```python
from build123d import *

# Parameters (mm, degrees)
SKETCH1_R            = 25
BOSS_EXTRUDE2_DEPTH  = 3
SKETCH3_R            = 57
BOSS_EXTRUDE10_DEPTH = 2
SKETCH8_R            = 51
SKETCH8_R_2          = 45
BOSS_EXTRUDE11_DEPTH = 6
SKETCH9_R            = 10
BOSS_EXTRUDE12_DEPTH = 6
SKETCH10_R           = 57
BOSS_EXTRUDE13_DEPTH = 2
FILLET1_R            = 2
FILLET2_R            = 2
FILLET3_R            = 2
FILLET4_R            = 2
SKETCH11_R           = 50
BOSS_EXTRUDE14_DEPTH = 10
CUT_EXTRUDE3_DEPTH   = 10


with BuildPart() as part:
    # Sketch1 → Boss-Extrude2 (new body)
    with BuildSketch(Plane(origin=(0, 0, 0), x_dir=(1, 0, 0), z_dir=(0, 1, 0))):
        Circle(SKETCH1_R)
        with BuildLine():
            Line((20, -3.5), (7.537849637, -5))
            ThreePointArc((7.537849637, -5), (6.396060395, -6.396060395), (5, -7.537849637))
            Line((5, -7.537849637), (3.5, -20))
            Line((3.5, -20), (-3.5, -20))
            Line((-3.5, -20), (-5, -7.537849637))
            ThreePointArc((-5, -7.537849637), (-6.396060395, -6.396060395), (-7.537849637, -5))
            Line((-7.537849637, -5), (-20, -3.5))
            Line((-20, -3.5), (-20, 3.5))
            Line((-20, 3.5), (-7.537849637, 5))
            ThreePointArc((-7.537849637, 5), (-6.396060395, 6.396060395), (-5, 7.537849637))
            Line((-5, 7.537849637), (-3.5, 20))
            Line((-3.5, 20), (3.5, 20))
            Line((3.5, 20), (5, 7.537849637))
            ThreePointArc((5, 7.537849637), (6.396060395, 6.396060395), (7.537849637, 5))
            Line((7.537849637, 5), (20, 3.5))
            Line((20, 3.5), (20, -3.5))
        make_face(mode=Mode.SUBTRACT)
    extrude(amount=BOSS_EXTRUDE2_DEPTH)

    # Sketch3 → Boss-Extrude10 (add)
    with BuildSketch(Plane(origin=(0, 3, 0), x_dir=(1, 0, 0), z_dir=(0, 1, 0))):
        Circle(SKETCH3_R)
    extrude(amount=BOSS_EXTRUDE10_DEPTH)

    # Sketch8 → Boss-Extrude11 (add)
    with BuildSketch(Plane(origin=(0, 5, 0), x_dir=(1, 0, 0), z_dir=(0, 1, 0))):
        Circle(SKETCH8_R)
        Circle(SKETCH8_R_2, mode=Mode.SUBTRACT)
    extrude(amount=BOSS_EXTRUDE11_DEPTH)

    # Sketch9 → Boss-Extrude12 (add)
    with BuildSketch(Plane(origin=(0, 5, 0), x_dir=(1, 0, 0), z_dir=(0, 1, 0))):
        Circle(SKETCH9_R)
    extrude(amount=BOSS_EXTRUDE12_DEPTH)

    # Sketch10 → Boss-Extrude13 (add)
    with BuildSketch(Plane(origin=(0, 11, 0), x_dir=(1, 0, 0), z_dir=(0, 1, 0))):
        Circle(SKETCH10_R)
    extrude(amount=BOSS_EXTRUDE13_DEPTH)

    # Fillet1
    fillet1_edges = [part.edges().sort_by_distance(p)[0] for p in [
        (-51, 11, 0),
    ]]
    fillet(fillet1_edges, radius=FILLET1_R)

    # Fillet2
    fillet2_edges = [part.edges().sort_by_distance(p)[0] for p in [
        (-51, 5, 0),
    ]]
    fillet(fillet2_edges, radius=FILLET2_R)

    # Fillet3
    fillet3_edges = [part.edges().sort_by_distance(p)[0] for p in [
        (-25, 3, 0),
    ]]
    fillet(fillet3_edges, radius=FILLET3_R)

    # Fillet4
    fillet4_edges = [part.edges().sort_by_distance(p)[0] for p in [
        (-25, 0, 0),
    ]]
    fillet(fillet4_edges, radius=FILLET4_R)

    # Sketch11 → Boss-Extrude14 (add)
    with BuildSketch(Plane(origin=(0, 13, 0), x_dir=(1, 0, 0), z_dir=(0, 1, 0))):
        Circle(SKETCH11_R)
    extrude(amount=-BOSS_EXTRUDE14_DEPTH)

    # Sketch12 → Cut-Extrude3 (cut)
    with BuildSketch(Plane(origin=(0, 13, 0), x_dir=(1, 0, 0), z_dir=(0, 1, 0))):
        with BuildLine():
            Line((44.129475009, -5), (5, -5))
            Line((5, -5), (5, -44.129475009))
            ThreePointArc((5, -44.129475009), (31.403905526, -31.403905526), (44.129475009, -5))
        make_face()
        with BuildLine():
            Line((5, 5), (44.129475009, 5))
            ThreePointArc((44.129475009, 5), (31.403905526, 31.403905526), (5, 44.129475009))
            Line((5, 44.129475009), (5, 5))
        make_face()
        with BuildLine():
            Line((-44.129475009, 5), (-5, 5))
            Line((-5, 5), (-5, 44.129475009))
            ThreePointArc((-5, 44.129475009), (-31.403905526, 31.403905526), (-44.129475009, 5))
        make_face()
        with BuildLine():
            Line((-5, -44.129475009), (-5, -5))
            Line((-5, -5), (-44.129475009, -5))
            ThreePointArc((-44.129475009, -5), (-31.403905526, -31.403905526), (-5, -44.129475009))
        make_face()
    extrude(amount=-CUT_EXTRUDE3_DEPTH, mode=Mode.SUBTRACT)


solid = part.part
```
CAD build for the part. Positions are in the model's coordinates, mm. A direction names the side the tool comes from. Give positions to 0.01 mm unless a question says otherwise; leave off trailing zeros.
(1) Saw through at A-A, the plane z = 31. State how many separate pieces and enclosed holes the cut face has, then the cut area to 3 significant figures.
(2) Drill centre lines: L1, parallel to X at y = 7.25, z = -36.5; L2, parallel to X at y = 4.5, z = 38.5; L3, parallel to Z at x = -33.5, y = 6. Where is each one in solid material? Low to high.
(3) Mould opens along X. For faces 4 (the cylindrical face through (-6.41, 1.48, -6.38)), 5 (the flat face through (38, 11, 38)) say: released by +X, released by -X, zero draft, split by the parting line, or undercut.
(4) Flat gauge pins, fed straight in: pin 1 (5 mm diameter, centred on x = 4, z = -25, fed in from -Y); pin 2 (1 mm diameter, centred on x = -3, y = 8, fed in from +Z); pin 3 (5 mm diameter, centred on y = 11, z = -23, fed in from -X); pin 4 (0.9 mm diameter, centred on x = 1, y = 1, fed in from -Z). Where does each tip first touch, or does it go through?
(5) Tool access for faces 1 (the flat face through (-14, 3, 13)), 2 (the flat face through (-13.68, 1.48, 4.26)), 3 (the cylindrical face through (-31.107, 8.07, -31.698)): list every direction of +Z, -Z, +X, -X, +Y, -Y with a clear straight run to the whole face (end or side of a thin tool).
Results found:
1. separate pieces: 3
1. enclosed holes: 0
1. area: 337 mm2
2. L1: x = -35.62 to -25.3, -5 to 5, 25.3 to 35.62
2. L2: x = -42.03 to -22.14, -5 to 5, 22.14 to 42.03
2. L3: z = -38.81 to -29.16, -5 to 5, 29.16 to 38.81
3. face 4: undercut
3. face 5: zero draft
4. pin 1: stops at y = 0
4. pin 2: stops at z = 50.94
4. pin 3: stops at x = -53.19
4. pin 4: stops at z = -25.03
5. face 1: +Y
5. face 2: -Y
5. face 3: +Y, -Y
